from build123d import *

# Parameters (mm, degrees)
SKETCH1_W           = 12
SKETCH1_H           = 16
SKETCH1_R           = 2.1
SKETCH1_W_2         = 2
BOSS_EXTRUDE1_DEPTH = 21
FILLET1_R           = 5
SKETCH2_W           = 9
SKETCH2_H           = 1.9
BOSS_EXTRUDE2_DEPTH = 5
SKETCH4_W           = 12
SKETCH4_H           = 21
BOSS_EXTRUDE3_DEPTH = 10.5
FILLET2_R           = 5.1
FILLET4_R           = 2
SKETCH6_W           = 3
SKETCH6_H           = 8
BOSS_EXTRUDE5_DEPTH = 8
FILLET6_R           = 2
FILLET8_R           = 5
BOSS_EXTRUDE6_DEPTH = 10
FILLET9_R           = 5


with BuildPart() as part:
    # Sketch1 → Boss-Extrude1 (new body)
    # profile 1 of 2: a face of its own
    with BuildSketch(Plane(origin=(0, 0, 0), x_dir=(1, 0, 0), z_dir=(0, 1, 0))):
        Rectangle(SKETCH1_W, SKETCH1_H)
        with Locations(Location((0, 0, 0), (0, 0, 90))):
            Circle(SKETCH1_R, mode=Mode.SUBTRACT)
    # profile 2 of 2: a face of its own
    with BuildSketch(Plane(origin=(0, 0, 0), x_dir=(1, 0, 0), z_dir=(0, 1, 0))):
        with Locations((7, 0)):
            Rectangle(SKETCH1_W_2, SKETCH1_H)
    extrude(amount=BOSS_EXTRUDE1_DEPTH)

    # Fillet1
    fillet1_edges = [part.edges().sort_by_distance(p)[0] for p in [
        (-6, 10.5, 8),
        (-6, 10.5, -8),
    ]]
    fillet(fillet1_edges, radius=FILLET1_R)

    # Sketch2 → Boss-Extrude2 (add)
    with BuildSketch(Plane(origin=(0, 21, 0), x_dir=(1, 0, 0), z_dir=(0, 1, 0))):
        with Locations((3.5, 7.05)):
            Rectangle(SKETCH2_W, SKETCH2_H)
        with Locations((3.5, -7.05)):
            Rectangle(SKETCH2_W, SKETCH2_H)
    extrude(amount=BOSS_EXTRUDE2_DEPTH)

    # Sketch4 → Boss-Extrude3 (add)
    with BuildSketch(Plane(origin=(8, 0, 0), x_dir=(0, 0, -1), z_dir=(1, 0, 0))):
        with Locations((0, 10.5)):
            Rectangle(SKETCH4_W, SKETCH4_H)
    extrude(amount=BOSS_EXTRUDE3_DEPTH)

    # Fillet2
    fillet2_edges = [part.edges().sort_by_distance(p)[0] for p in [
        (18.5, 21, 0),
    ]]
    fillet(fillet2_edges, radius=FILLET2_R)

    # Fillet4
    fillet4_edges = [part.edges().sort_by_distance(p)[0] for p in [
        (-1, 21, -7.05),
        (-1, 21, 7.05),
        (8, 10.5, -6),
        (8, 10.5, 6),
    ]]
    fillet(fillet4_edges, radius=FILLET4_R - 0.0001)  # a hair under: the kernel refuses the full size

    # Sketch6 → Boss-Extrude5 (add)
    with BuildSketch(Plane.XZ):
        with Locations((11.6, 0)):
            Rectangle(SKETCH6_W, SKETCH6_H)
    extrude(amount=BOSS_EXTRUDE5_DEPTH)

    # Fillet6
    fillet6_edges = [part.edges().sort_by_distance(p)[0] for p in [
        (11.6, 0, -4),
        (11.6, 0, 4),
    ]]
    fillet(fillet6_edges, radius=FILLET6_R - 0.0001)  # a hair under: the kernel refuses the full size

    # Fillet8
    fillet8_edges = [part.edges().sort_by_distance(p)[0] for p in [
        (13.1, 0, 0),
    ]]
    fillet(fillet8_edges, radius=FILLET8_R)

    # Sketch7 → Boss-Extrude6 (add)
    with BuildSketch(Plane(origin=(18.5, 0, 0), x_dir=(0, 0, -1), z_dir=(1, 0, 0))):
        Polygon((-6, 0), (-6, 6.45), (6, 7.078893351), (6, 0), align=None)
    extrude(amount=BOSS_EXTRUDE6_DEPTH)

    # Fillet9
    fillet9_edges = [part.edges().sort_by_distance(p)[0] for p in [
        (28.5, 0, 0),
    ]]
    fillet(fillet9_edges, radius=FILLET9_R)


solid = part.part
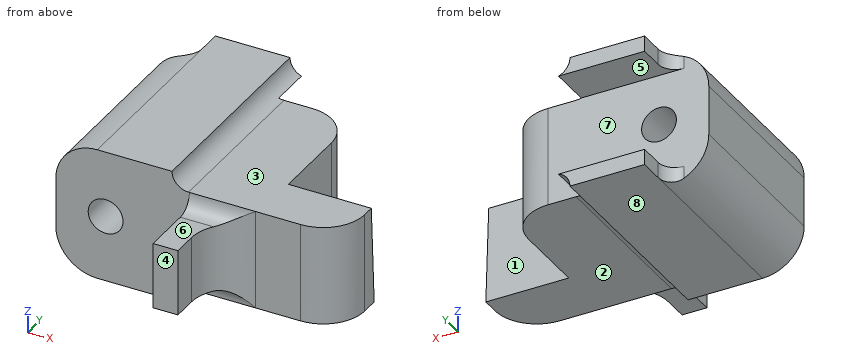
Read the model definition and answer for the solid it produces. Units are mm, in the model's axes. Face numbers are marked on the shaded views. A direction names the side the tool comes from. Round coordinates to 2 decimals unless told otherwise and drop trailing zeros. Write each loop counter-clockwise with the first axis right and the second up, starting at its lowest first coordinate (ties: lowest second). Pieces come first, ordered by that corner, then holes.
Q1. A tool of negligible diameter and unlimited length cuts with its end or side. For the marked faces 1, 2, 3, 4 and 5, from which of +Z, -Z, +X, -X, +Y, -Y can it reach the whole face along a straight path? Write none if from no direction.
Values:
face 1: +Z, +X, +Y
face 2: -Z, +X, +Y, -Y
face 3: +Z, +X, +Y, -Y
face 4: +Z, -Z, +X, -X, -Y
face 5: +X, -X, +Y
Q2. Find section B-B on z = -1. Determine the outline of the cut face in (x, y).
Values:
outline: (-6, 0) - (-1.85, 0) - (-1.85, 21) - (-6, 21) - close; (1.85, 0) - (10.1, 0) - (10.1, -8) - (13.1, -8) - (13.1, -5) arc R5 cw to (18.1, 0) - (23.5, 0) arc R5 ccw to (28.5, 5) - (28.5, 6.82) - (18.5, 6.82) - (18.5, 15.9) arc R5.1 ccw to (13.4, 21) - (1.85, 21) - close
Q3. The mould has two halves that part along Z. Classify the marked faces 6, 7 and 8: released by +Z, released by -Z, zero draft, split by the parting line, or undercut.
Values:
face 6: released by +Z
face 7: undercut
face 8: released by -Z
Q4. Flat-ended cylindrical pins translate along their axes: P1, Ø5, axis at x = 24.5, z = -3.5, coming from the -Y side; P2, Ø10, axis at x = 16, y = -3, coming from the +Z side; P3, Ø4.5, axis at x = 11, y = -4, coming from the +Z side. Find the tip coordinate at first contact, or state that the pin passes through.
Values:
P1: stops at y = 0
P2: stops at z = 6
P3: stops at z = 4.02
Q5. Find section C-C on x = 20. Determine the outline of the cut face in (y, z), and give its area (3 significant figures).
Values:
outline: (0, -6) - (7.08, -6) - (6.45, 6) - (0, 6) - close
area: 81.2 mm2
